```python
from build123d import *

# Parameters (mm, degrees)
F0_W     = 2.375
F0_H     = 19.5291
F1_DEPTH = 1000
F2_R     = 2.2479
F3_DEPTH = 4.75


with BuildPart() as f1:
    # F0 (on Top) → F1 (new body)
    with BuildSketch(Plane.XY):
        with BuildLine():
            Line((0, 0.921682), (0, 0))
            Line((0, 0), (2.375, 0))
            Line((2.375, 0), (4.75, 0))
            Line((4.75, 0), (4.75, 0.921682))
            Line((4.75, 0.921682), (2.936266, 2.735416))
            ThreePointArc((2.936266, 2.735416), (2.375, 2.9679), (1.813734, 2.735416))
            Line((1.813734, 2.735416), (0, 0.921682))
        make_face()
        with Locations((1.1875, -9.76455)):
            Rectangle(F0_W, F0_H)
    extrude(amount=F1_DEPTH)

    # F2 (on face) → F3 (cut, through all)
    with BuildSketch(Plane(origin=(0, 0, 0), x_dir=(0, -1, 0), z_dir=(-1, 0, 0))):
        Polygon((19.5291, 898.24813), (19.5291, 1000), (1.5875, 1000), align=None)
        with Locations((5.55625, 777.007047)):
            Circle(F2_R)
        with Locations((5.55625, 532.532047)):
            Circle(F2_R)
    extrude(amount=-F3_DEPTH, mode=Mode.SUBTRACT)


solid = f1.part
```
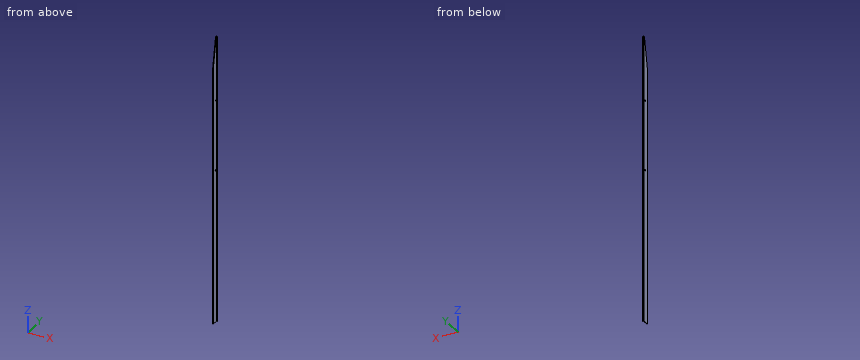
Input: part model. Units: mm. Frame: model coordinates. Give positions to 0.01 mm unless a question says otherwise; leave off trailing zeros. Write each loop counter-clockwise with the first axis right and the second up, starting at its lowest first coordinate (ties: lowest second). Pieces come first, ordered by that corner, then holes. Notation, with made-up numbers: (26.25, 13.5) - (73.25, 13.5) arc R26 cw to (73.25, 38.5) - close; hole circle Ø7 at (76.5, -17.75). An arc over 180 degrees is marked (long way). Write item = value, one per line. Start each with the question number.
1. Ray query, L1, parallel to Y at x = 2.3, z = 783; L2, parallel to Y at x = 2, z = 432.5; L3, parallel to X at y = -13.75, z = 326 (3 decimals). Return the intervals inside material, ascending.
2. Section query C-C, the plane y = -12.5. Output: boundary loops of the cut face in (x, z) (3 decimals), then the cut area to 3 significant figures.
3. First-contact query: pin 1 Ø6 at (y, z) = (-14, 469) entering from +X (3 decimals); pin 2 Ø1.2 at (x, z) = (4, 647) entering from -Y. Flat tips, straight axial feed; report the tip coordinate or a pass-through.
4. Section query A-A, the plane x = 0.9. Output: boundary loops of the cut face in (y, z), then the cut area to 3 significant figures.
Check sheet entries:
q1.L1 = -19.53 to 2.96
q1.L2 = -19.53 to 2.87
q1.L3 = 0 to 2.375
q2.outline = (0, 0) - (2.375, 0) - (2.375, 938.112) - (0, 938.112) - close
q2.area = 2,230 mm2
q3.pin_1 = 2.375
q3.pin_2 = 0
q4.outline = (-19.53, 0) - (1.82, 0) - (1.82, 1000) - (-1.59, 1000) - (-19.53, 898.25) - close; hole circle Ø4.5 at (-5.56, 532.53); hole circle Ø4.5 at (-5.56, 777.01)
q4.area = 20,400 mm2
